from build123d import *

# Parameters (mm, degrees)
SKETCH_1_W      = 70
SKETCH_1_H      = 50
EXTRUDE_1_DEPTH = 10
EXTRUDE_2_DEPTH = 15


with BuildPart() as part:
    # 草图1 → 凸台-拉伸1 (new, symmetric)
    with BuildSketch(Plane.XY):
        Rectangle(SKETCH_1_W, SKETCH_1_H)
    extrude(amount=EXTRUDE_1_DEPTH, both=True)

    # 草图2 → 凸台-拉伸2 (add)
    with BuildSketch(Plane.XY.offset(10)):
        Polygon((12, 0), (-6, 10.392304845), (-6, -10.392304845), align=None)
    extrude(amount=EXTRUDE_2_DEPTH)


solid = part.part
Input: part model. Units: mm. Frame: model coordinates. A direction names the side the tool comes from. Coordinates: 2 decimals unless noted, no trailing zeros. Loops run counter-clockwise (first coordinate to the right, second up) from the corner with the lowest first, then second, coordinate; pieces in that order, holes last.
Q1. Material intervals for line 1 (Z direction, x = 4, y = 22); line 2 (Y direction, x = 7, z = 19.5); line 3 (X direction, y = 5, z = 14), sorted ascending.
Q2. Cut plane D-D (y = 3). Output: boundary loops of the cut face in (x, z), then the cut area to 3 significant figures.
Q3. Cut plane A-A (y = -5). Output: boundary loops of the cut face in (x, z).
Q4. Contact query for flat-ended pins moving along their axis: pin 1 (8 mm diameter, centred on y = 15.5, z = 20.5, fed in from +X); pin 2 (12 mm diameter, centred on y = -4, z = 20, fed in from -X). Output: stop coordinate, or through.
Q5. Set-up query: faces 1 (the face through (-6, 0, 17)), 2 (the face through (1, 0, 25)), 3 (the face through (0, 25, 0)), 4 (the face through (2.87, -5.27, 17.4)), 5 (the face through (3.13, 5.12, 17.4)). Return all of +Z, -Z, +X, -X, +Y, -Y with unobstructed straight access to the full face (end or side cutting, diameter ignored); none if empty.
Q6. Cut plane B-B (x = 29.5). Output: boundary loops of the cut face in (y, z), then the cut area to 3 significant figures.
Q7. Cut plane C-C (z = 21). Output: boundary loops of the cut face in (x, y).
Working result:
1. line 1: z = -10 to 10
1. line 2: y = -2.89 to 2.89
1. line 3: x = -6 to 3.34
2. outline: (-35, -10) - (35, -10) - (35, 10) - (6.8, 10) - (6.8, 25) - (-6, 25) - (-6, 10) - (-35, 10) - close
2. area: 1,590 mm2
3. outline: (-35, -10) - (35, -10) - (35, 10) - (3.34, 10) - (3.34, 25) - (-6, 25) - (-6, 10) - (-35, 10) - close
4. pin 1: passes through
4. pin 2: stops at x = -6
5. face 1: +Z, -X, +Y, -Y
5. face 2: +Z, +X, -X, +Y, -Y
5. face 3: +Z, -Z, +X, -X, +Y
5. face 4: +Z, +X, -Y
5. face 5: +Z, +X, +Y
6. outline: (-25, -10) - (25, -10) - (25, 10) - (-25, 10) - close
6. area: 1,000 mm2
7. outline: (-6, -10.39) - (12, 0) - (-6, 10.39) - close
